Here's how the part is built. I have some questions about the finished solid (model axes, mm). A direction names the side the tool comes from. Round coordinates to 2 decimals unless told otherwise and drop trailing zeros. Loops run counter-clockwise (first coordinate to the right, second up) from the corner with the lowest first, then second, coordinate; pieces in that order, holes last. Notation, with made-up numbers: (27.5, 10) - (51.5, 10) arc R34 ccw to (51.5, 40) - close; hole circle Ø1 at (-32, -20). An arc over 180 degrees is marked (long way). Return JSON: item names as keys, results as strings. Group by question number.
```python
from build123d import *

# Parameters (mm, degrees)
SKETCH_1_W          = 100
SKETCH_1_H          = 100
SKETCH_1_R          = 1.5
EXTRUDE_1_DEPTH     = 3
SKETCH_4_W          = 100
SKETCH_4_H          = 100
EXTRUDE_4_DEPTH     = 23
SKETCH_5_R          = 4
SKETCH_5_R_2        = 1.5
EXTRUDE_5_DEPTH     = 13
FILLET_2_R          = 2
FILLET_3_R          = 8
SKETCH_7_R          = 1.5
EXTRUDE_6_DEPTH     = 23
SKETCH_8_R          = 1.75
SKETCH_8_R_2        = 2
CUT_EXTRUDE_2_DEPTH = 3


with BuildPart() as part:
    # Эскиз1 → Бобышка-Вытянуть1 (new body)
    with BuildSketch(Plane(origin=(0, 0, 0), x_dir=(1, 0, 0), z_dir=(0, 1, 0))):
        with Locations((50, 50)):
            Rectangle(SKETCH_1_W, SKETCH_1_H)
        with Locations(Location((14.7, 81, 0), (0, 0, 270))):
            Circle(SKETCH_1_R, mode=Mode.SUBTRACT)
        with Locations(Location((71.7, 75, 0), (0, 0, 270))):
            Circle(SKETCH_1_R, mode=Mode.SUBTRACT)
        with Locations(Location((71.7, 25, 0), (0, 0, 90))):
            Circle(SKETCH_1_R, mode=Mode.SUBTRACT)
        with Locations(Location((14.7, 19, 0), (0, 0, 90))):
            Circle(SKETCH_1_R, mode=Mode.SUBTRACT)
        with Locations(Location((7, 93, 0), (0, 0, 270))):
            Circle(SKETCH_1_R, mode=Mode.SUBTRACT)
        with Locations(Location((93, 93, 0), (0, 0, 90))):
            Circle(SKETCH_1_R, mode=Mode.SUBTRACT)
        with Locations(Location((93, 7, 0), (0, 0, 270))):
            Circle(SKETCH_1_R, mode=Mode.SUBTRACT)
        with Locations(Location((7, 7, 0), (0, 0, 90))):
            Circle(SKETCH_1_R, mode=Mode.SUBTRACT)
    extrude(amount=EXTRUDE_1_DEPTH)

    # Эскиз4 → Бобышка-Вытянуть4 (add)
    with BuildSketch(Plane(origin=(0, 3, 0), x_dir=(1, 0, 0), z_dir=(0, 1, 0))):
        with Locations((50, 50)):
            Rectangle(SKETCH_4_W, SKETCH_4_H)
        with BuildLine():
            Line((97, 97), (3, 97))
            Line((3, 97), (3, 65.304901176))
            ThreePointArc((3, 65.304901176), (2.879271228, 63.755707837), (2.52, 62.243920941))
            ThreePointArc((2.52, 62.243920941), (0.6, 50), (2.52, 37.756079059))
            ThreePointArc((2.52, 37.756079059), (2.879271228, 36.244292163), (3, 34.695098824))
            Line((3, 34.695098824), (3, 3))
            Line((3, 3), (97, 3))
            Line((97, 3), (97, 37.262653338))
            ThreePointArc((97, 37.262653338), (97.172923702, 39.114293537), (97.685714286, 40.901895241))
            ThreePointArc((97.685714286, 40.901895241), (99.4, 50), (97.685714286, 59.098104759))
            ThreePointArc((97.685714286, 59.098104759), (97.172923702, 60.885706463), (97, 62.737346662))
            Line((97, 62.737346662), (97, 97))
        make_face(mode=Mode.SUBTRACT)
    extrude(amount=EXTRUDE_4_DEPTH)

    # Эскиз5 → Бобышка-Вытянуть5 (add)
    # profile 1 of 4: a face of its own
    with BuildSketch(Plane(origin=(0, 3, 0), x_dir=(1, 0, 0), z_dir=(0, 1, 0))):
        with Locations(Location((14.7, 81, 0), (0, 0, 90))):
            Circle(SKETCH_5_R)
        with Locations(Location((14.7, 81, 0), (0, 0, 270))):
            Circle(SKETCH_5_R_2, mode=Mode.SUBTRACT)
    # profile 2 of 4: a face of its own
    with BuildSketch(Plane(origin=(0, 3, 0), x_dir=(1, 0, 0), z_dir=(0, 1, 0))):
        with Locations(Location((71.7, 75, 0), (0, 0, 90))):
            Circle(SKETCH_5_R)
        with Locations(Location((71.7, 75, 0), (0, 0, 270))):
            Circle(SKETCH_5_R_2, mode=Mode.SUBTRACT)
    # profile 3 of 4: a face of its own
    with BuildSketch(Plane(origin=(0, 3, 0), x_dir=(1, 0, 0), z_dir=(0, 1, 0))):
        with Locations(Location((71.7, 25, 0), (0, 0, 90))):
            Circle(SKETCH_5_R)
        with Locations(Location((71.7, 25, 0), (0, 0, 90))):
            Circle(SKETCH_5_R_2, mode=Mode.SUBTRACT)
    # profile 4 of 4: a face of its own
    with BuildSketch(Plane(origin=(0, 3, 0), x_dir=(1, 0, 0), z_dir=(0, 1, 0))):
        with Locations(Location((14.7, 19, 0), (0, 0, 90))):
            Circle(SKETCH_5_R)
        with Locations(Location((14.7, 19, 0), (0, 0, 90))):
            Circle(SKETCH_5_R_2, mode=Mode.SUBTRACT)
    extrude(amount=EXTRUDE_5_DEPTH)

    # Скругление2
    fillet_2_edges = [part.edges().sort_by_distance(p)[0] for p in [
        (71.7, 3, -21),
        (14.7, 3, -15),
        (14.7, 3, -77),
        (71.7, 3, -71),
    ]]
    fillet(fillet_2_edges, radius=FILLET_2_R)

    # Скругление3
    fillet_3_edges = [part.edges().sort_by_distance(p)[0] for p in [
        (0, 13, -100),
        (100, 13, -100),
        (100, 13, 0),
        (0, 13, 0),
    ]]
    fillet(fillet_3_edges, radius=FILLET_3_R)

    # Эскиз7 → Бобышка-Вытянуть6 (add)
    # profile 1 of 4: a face of its own
    with BuildSketch(Plane(origin=(0, 3, 0), x_dir=(1, 0, 0), z_dir=(0, 1, 0))):
        with BuildLine():
            Line((3, 89), (3, 97))
            Line((3, 97), (11, 97))
            Line((11, 97), (11, 93))
            ThreePointArc((11, 93), (9.828427125, 90.171572875), (7, 89))
            Line((7, 89), (3, 89))
        make_face()
        with Locations(Location((7, 93, 0), (0, 0, 270))):
            Circle(SKETCH_7_R, mode=Mode.SUBTRACT)
    # profile 2 of 4: a face of its own
    with BuildSketch(Plane(origin=(0, 3, 0), x_dir=(1, 0, 0), z_dir=(0, 1, 0))):
        with BuildLine():
            Line((89, 93), (89, 97))
            Line((89, 97), (97, 97))
            Line((97, 97), (97, 89))
            Line((97, 89), (93, 89))
            ThreePointArc((93, 89), (90.171572875, 90.171572875), (89, 93))
        make_face()
        with Locations(Location((93, 93, 0), (0, 0, 90))):
            Circle(SKETCH_7_R, mode=Mode.SUBTRACT)
    # profile 3 of 4: a face of its own
    with BuildSketch(Plane(origin=(0, 3, 0), x_dir=(1, 0, 0), z_dir=(0, 1, 0))):
        with BuildLine():
            Line((97, 11), (97, 3))
            Line((97, 3), (89, 3))
            Line((89, 3), (89, 7))
            ThreePointArc((89, 7), (90.171572875, 9.828427125), (93, 11))
            Line((93, 11), (97, 11))
        make_face()
        with Locations(Location((93, 7, 0), (0, 0, 270))):
            Circle(SKETCH_7_R, mode=Mode.SUBTRACT)
    # profile 4 of 4: a face of its own
    with BuildSketch(Plane(origin=(0, 3, 0), x_dir=(1, 0, 0), z_dir=(0, 1, 0))):
        with BuildLine():
            Line((11, 7), (11, 3))
            Line((11, 3), (3, 3))
            Line((3, 3), (3, 11))
            Line((3, 11), (7, 11))
            ThreePointArc((7, 11), (9.828427125, 9.828427125), (11, 7))
        make_face()
        with Locations(Location((7, 7, 0), (0, 0, 90))):
            Circle(SKETCH_7_R, mode=Mode.SUBTRACT)
    extrude(amount=EXTRUDE_6_DEPTH)

    # Эскиз8 → Вырез-Вытянуть2 (cut)
    with BuildSketch(Plane(origin=(0, 3, 0), x_dir=(1, 0, 0), z_dir=(0, 1, 0))):
        with Locations(Location((20, 90, 0), (0, 0, 270))):
            Circle(SKETCH_8_R)
        with Locations(Location((80, 90, 0), (0, 0, 90))):
            Circle(SKETCH_8_R)
        with Locations(Location((80, 10, 0), (0, 0, 270))):
            Circle(SKETCH_8_R)
        with Locations(Location((20, 10, 0), (0, 0, 90))):
            Circle(SKETCH_8_R)
        with Locations(Location((89.900400778, 61.508405751, 0), (0, 0, 270))):
            Circle(SKETCH_8_R_2)
        with Locations(Location((80, 61.508405751, 0), (0, 0, 270))):
            Circle(SKETCH_8_R_2)
        with BuildLine():
            Line((12.592071992, 57.5), (87.592071992, 57.5))
            ThreePointArc((87.592071992, 57.5), (95.092071992, 50), (87.592071992, 42.5))
            Line((87.592071992, 42.5), (12.592071992, 42.5))
            ThreePointArc((12.592071992, 42.5), (5.092071992, 50), (12.592071992, 57.5))
        make_face()
    extrude(amount=-CUT_EXTRUDE_2_DEPTH, mode=Mode.SUBTRACT)


solid = part.part
```
Q1. Imagine slicing it at D-D, the plane z = -39. List the corners of the cut face in (x, y) for me, and give its area (3 significant figures).
Q2. For faces 1 (the cylindrical face through (5.094, 1.521, -49.835)), 2 (the cylindrical face through (2.883, 14.339, -63.777)), 3 (the cylindrical face through (2.281, 12.818, -97.594)), which set-ups out of +Z, -Z, +X, -X, +Y, -Y let a thin tool reach every point of the face, with its end or its side?
Q3. Will these pins go through, and if not, where does the flat tip stop? pin 1 Ø1.2 at (y, z) = (20, -5.5) entering from +X; pin 2 Ø10 at (x, z) = (45.5, -32.5) entering from +Y; pin 3 Ø4 at (x, z) = (14, -20) entering from +Y; pin 4 Ø3 at (x, z) = (20, -10) entering from -Y.
Q4. Imagine slicing it at A-A, the plane x = 14.7. Give the number of separate pieces and of enclosed holes in the cut face, and give its area (3 significant figures).
Q5. Please list where these lines run through material, in increasing order: line 1 (X direction, y = 1.1, z = -90); line 2 (X direction, y = 7, z = -75); line 3 (X direction, y = 13.5, z = -94).
Q6. Imagine slicing it at B-B, the plane z = -50. List the corners of the cut face in (x, y) for me.
Q7. If we mould it in two halves opening along Z, with no side actions, what happens to faces 4 (the flat face through (49, 0, -62)), 5 (the cylindrical face through (97.594, 12.818, -97.719)), 6 (the flat face through (50, 2, -57.5))? For each: +Z half, -Z half, draft (parallel to the pull), parting line (faces both ways), or undercut.
Output values:
{
 "1": {"outline": "(0, 0) - (100, 0) - (100, 26) - (97.15, 26) - (97.15, 3) - (2.14, 3) - (2.14, 26) - (0, 26) - close", "area": "415 mm^2"},
 "2": {"face 1": "+Y, -Y", "face 2": "+Y", "face 3": "-Z, -X, +Y, -Y"},
 "3": {"pin 1": "stops at x = 99.77", "pin 2": "stops at y = 3", "pin 3": "stops at y = 16", "pin 4": "passes through"},
 "4": {"separate pieces": "4", "enclosed holes": "0", "area": "508 mm^2"},
 "5": {"line 1": "x = 0 to 18.25, 21.75 to 78.25, 81.75 to 100", "line 2": "x = 0 to 3, 67.7 to 70.2, 73.2 to 75.7, 97 to 100", "line 3": "x = 0.25 to 5.88, 8.12 to 11, 89 to 91.88, 94.12 to 99.75"},
 "6": {"outline": "(0, 0) - (5.09, 0) - (5.09, 3) - (0.6, 3) - (0.6, 26) - (0, 26) - close; (95.09, 0) - (100, 0) - (100, 26) - (99.4, 26) - (99.4, 3) - (95.09, 3) - close"},
 "7": {"face 4": "draft", "face 5": "-Z half", "face 6": "undercut"}
}
